Verification items for the finished model (mm, model axes). A direction names the side the tool comes from. Coordinates: 2 decimals unless noted, no trailing zeros. Write each loop counter-clockwise with the first axis right and the second up, starting at its lowest first coordinate (ties: lowest second). Pieces come first, ordered by that corner, then holes. Notation, with made-up numbers: (54.5, 52) -> (96.5, 52) arc R27 ccw to (96.5, 74) -> close; hole circle Ø6 at (-18.5, 11.25). An arc over 180 degrees is marked (long way). Answer in a Markdown table with one row per item.
```python
from build123d import *

# Parameters (mm, degrees)
SKETCH1_R             = 10
BOSS_EXTRUDE1_DEPTH   = 300
BOSS_EXTRUDE1_2_DEPTH = 300
BOSS_EXTRUDE1_3_DEPTH = 300
SKETCH1_3_R           = 150
BOSS_EXTRUDE2_DEPTH   = 10


with BuildPart() as part:
    # Sketch1 → Boss-Extrude1 (new body)
    with BuildSketch(Plane(origin=(0, 0, 0), x_dir=(1, 0, 0), z_dir=(0, 1, 0))):
        with Locations(Location((-150, 0, 0), (0, 0, 270))):
            Circle(SKETCH1_R)
    extrude(amount=BOSS_EXTRUDE1_DEPTH)



with BuildPart() as body_2:
    # Sketch1 → Boss-Extrude1 2 (new body)
    with BuildSketch(Plane(origin=(0, 0, 0), x_dir=(1, 0, 0), z_dir=(0, 1, 0))):
        with Locations(Location((75, 129.903810568, 0), (0, 0, 270))):
            Circle(SKETCH1_R)
    extrude(amount=BOSS_EXTRUDE1_2_DEPTH)


with BuildPart() as body_3:
    # Sketch1 → Boss-Extrude1 3 (new body)
    with BuildSketch(Plane(origin=(0, 0, 0), x_dir=(1, 0, 0), z_dir=(0, 1, 0))):
        with Locations(Location((75, -129.903810568, 0), (0, 0, 270))):
            Circle(SKETCH1_R)
    extrude(amount=BOSS_EXTRUDE1_3_DEPTH)


with BuildPart() as part_1:
    add(part.part)

    add(body_2.part)  # Boss-Extrude2 merges body 2

    add(body_3.part)  # Boss-Extrude2 merges body 3
    # Sketch1_3 → Boss-Extrude2 (add)
    with BuildSketch(Plane(origin=(0, 0, 0), x_dir=(1, 0, 0), z_dir=(0, 1, 0))):
        with Locations(Location((0, 0, 0), (0, 0, 270))):
            Circle(SKETCH1_3_R)
    extrude(amount=-BOSS_EXTRUDE2_DEPTH)


solid = part_1.part
```
1. Mould release check, pull along Z, two halves, no side actions. Record for faces 4 (the cylindrical face through (-159.76, 147.9, -2.17)), 5 (the cylindrical face through (84.915, 147.9, 128.602)), 6 (the flat face through (-154, 0, 0)): released by +Z, released by -Z, zero draft, split by the parting line, or undercut.
Geometry says:
| item | result |
|---|---|
| face 4 | split by the parting line |
| face 5 | undercut |
| face 6 | zero draft |
2. Section check C-C, the plane x = 16.5. Record the boundary of the cut face in (y, z), plus the area to 3 significant figures.
Geometry says:
| item | result |
|---|---|
| outline | (-10, -149.09) -> (0, -149.09) -> (0, 149.09) -> (-10, 149.09) -> close |
| area | 2,980 mm^2 |
3. Depth check by flat-ended pin: P1, Ø8.5, axis at x = -156.5, z = 1, coming from the -Y side; P2, Ø7.5, axis at x = 80.5, z = 129, coming from the -Y side; P3, Ø6, axis at x = -66, z = -64.5, coming from the +Y side. Enter the tip coordinate at first touch or a pass-through.
Geometry says:
| item | result |
|---|---|
| P1 | y = 0 |
| P2 | y = -10 |
| P3 | y = 0 |
4. Section check A-A, the plane z = 0. Record the boundary of the cut face in (x, y), plus the area to 3 significant figures.
Geometry says:
| item | result |
|---|---|
| outline | (-160, 0) -> (-150, 0) -> (-150, -10) -> (150, -10) -> (150, 0) -> (-140, 0) -> (-140, 300) -> (-160, 300) -> close |
| area | 9,000 mm^2 |
5. Thickness scan on line 1 (Y direction, x = 120, z = 87); line 2 (Z direction, x = -142, y = 38); line 3 (X direction, y = 42.5, z = 125). Record the ranges inside material, lowest first. Write a range as from..to.
Geometry says:
| item | result |
|---|---|
| line 1 | -10..0 |
| line 2 | -6..6 |
| line 3 | 66.28..83.72 |
6. Tool access check on faces 1 (the cylindrical face through (78.004, 147.9, -120.366)), 2 (the flat face through (78, 0, -134)), 3 (the flat face through (2, -10, -2)). Record the directions out of +Z, -Z, +X, -X, +Y, -Y that give a thin tool (end or side, any length) a straight path to the whole face; none if there is none.
Geometry says:
| item | result |
|---|---|
| face 1 | +Y |
| face 2 | -Z, +X, -Y |
| face 3 | +Z, -Z, +X, -X, -Y |
7. Section check D-D, the plane z = 83.5. Record the boundary of the cut face in (x, y), plus the area to 3 significant figures.
Geometry says:
| item | result |
|---|---|
| outline | (-124.61, -10) -> (124.61, -10) -> (124.61, 0) -> (-124.61, 0) -> close |
| area | 2,490 mm^2 |
8. Section check B-B, the plane y = 110.5. Record the boundary of the cut face in (x, z), plus the area to 3 significant figures.
Geometry says:
| item | result |
|---|---|
| outline | circle Ø20 at (-150, 0); circle Ø20 at (75, -129.9); circle Ø20 at (75, 129.9) |
| area | 942 mm^2 |
